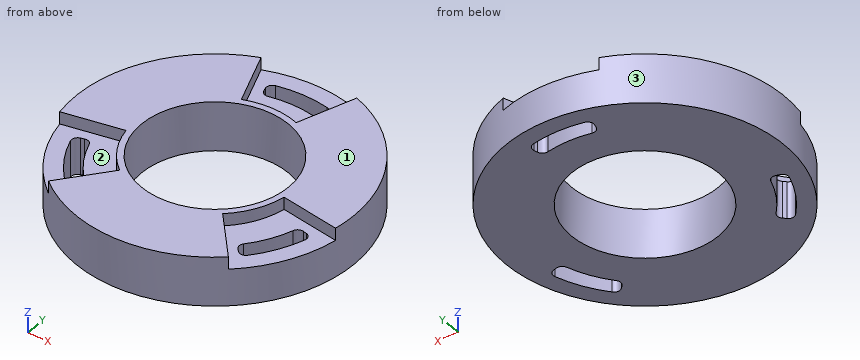
from build123d import *

# Parameters (mm, degrees)
CROQUIS1_R              = 11.35
CROQUIS1_R_2            = 6
SALIENTE_EXTRUIR1_DEPTH = 4
CORTAR_EXTRUIR1_START   = -1
CORTAR_EXTRUIR1_DEPTH   = 1


with BuildPart() as part:
    # Croquis1 → Saliente-Extruir1 (new body)
    with BuildSketch(Plane.XY):
        Circle(CROQUIS1_R)
        Circle(CROQUIS1_R_2, mode=Mode.SUBTRACT)
        with BuildLine():
            Line((2.377616051, 8.873383904), (2.455373053, 9.163576986))
            ThreePointArc((2.455373053, 9.163576986), (2.398691549, 9.55429889), (2.0762212, 9.782091061))
            ThreePointArc((2.0762212, 9.782091061), (0, 10), (-2.0762212, 9.782091061))
            ThreePointArc((-2.0762212, 9.782091061), (-2.398691549, 9.55429889), (-2.455373053, 9.163576986))
            Line((-2.455373053, 9.163576986), (-2.377616051, 8.873383904))
            ThreePointArc((-2.377616051, 8.873383904), (-2.15633175, 8.576736735), (-1.791682859, 8.513511175))
            ThreePointArc((-1.791682859, 8.513511175), (0, 8.7), (1.791682859, 8.513511175))
            ThreePointArc((1.791682859, 8.513511175), (2.15633175, 8.576736735), (2.377616051, 8.873383904))
        make_face(mode=Mode.SUBTRACT)
        with BuildLine():
            Line((8.873383904, -2.377616051), (9.163576986, -2.455373053))
            ThreePointArc((9.163576986, -2.455373053), (9.473611328, -2.699821628), (9.509649961, -3.092985228))
            ThreePointArc((9.509649961, -3.092985228), (8.660254038, -5), (7.433428761, -6.689105834))
            ThreePointArc((7.433428761, -6.689105834), (7.074919779, -6.854477262), (6.708203932, -6.708203932))
            Line((6.708203932, -6.708203932), (6.495767853, -6.495767853))
            ThreePointArc((6.495767853, -6.495767853), (6.34950602, -6.155806442), (6.477075524, -5.808398459))
            ThreePointArc((6.477075524, -5.808398459), (7.534421013, -4.35), (8.268758383, -2.705112716))
            ThreePointArc((8.268758383, -2.705112716), (8.505837769, -2.420930294), (8.873383904, -2.377616051))
        make_face(mode=Mode.SUBTRACT)
        with BuildLine():
            Line((-6.495767853, -6.495767853), (-6.708203932, -6.708203932))
            ThreePointArc((-6.708203932, -6.708203932), (-7.074919779, -6.854477262), (-7.433428761, -6.689105834))
            ThreePointArc((-7.433428761, -6.689105834), (-8.660254038, -5), (-9.509649961, -3.092985228))
            ThreePointArc((-9.509649961, -3.092985228), (-9.473611328, -2.699821628), (-9.163576986, -2.455373053))
            Line((-9.163576986, -2.455373053), (-8.873383904, -2.377616051))
            ThreePointArc((-8.873383904, -2.377616051), (-8.505837769, -2.420930294), (-8.268758383, -2.705112716))
            ThreePointArc((-8.268758383, -2.705112716), (-7.534421013, -4.35), (-6.477075524, -5.808398459))
            ThreePointArc((-6.477075524, -5.808398459), (-6.34950602, -6.155806442), (-6.495767853, -6.495767853))
        make_face(mode=Mode.SUBTRACT)
    extrude(amount=SALIENTE_EXTRUIR1_DEPTH)

    # Croquis2 → Cortar-Extruir1 (cut)
    with BuildSketch(Plane.XY.offset(4).offset(CORTAR_EXTRUIR1_START)):
        with BuildLine():
            Line((2.223130932, 6.108002035), (3.881928627, 10.665511246))
            ThreePointArc((3.881928627, 10.665511246), (0, 11.35), (-3.881928627, 10.665511246))
            Line((-3.881928627, 10.665511246), (-2.223130932, 6.108002035))
            ThreePointArc((-2.223130932, 6.108002035), (0, 6.5), (2.223130932, 6.108002035))
        make_face()
        with BuildLine():
            Line((6.401250395, -1.128713155), (11.177567997, -1.970906817))
            ThreePointArc((11.177567997, -1.970906817), (9.829388333, -5.675), (7.29563937, -8.694604429))
            Line((7.29563937, -8.694604429), (4.178119463, -4.97928888))
            ThreePointArc((4.178119463, -4.97928888), (5.629165125, -3.25), (6.401250395, -1.128713155))
        make_face()
        with BuildLine():
            Line((-4.178119463, -4.97928888), (-7.29563937, -8.694604429))
            ThreePointArc((-7.29563937, -8.694604429), (-9.829388333, -5.675), (-11.177567997, -1.970906817))
            Line((-11.177567997, -1.970906817), (-6.401250395, -1.128713155))
            ThreePointArc((-6.401250395, -1.128713155), (-5.629165125, -3.25), (-4.178119463, -4.97928888))
        make_face()
    extrude(amount=CORTAR_EXTRUIR1_DEPTH, mode=Mode.SUBTRACT)


solid = part.part
The listing builds one solid part. Answer for the finished solid, in the listing's coordinates (mm). Face numbers are marked on the shaded views. Coordinates: 2 decimals unless noted, no trailing zeros. Write each loop counter-clockwise with the first axis right and the second up, starting at its lowest first coordinate (ties: lowest second). Pieces come first, ordered by that corner, then holes. Notation, with made-up numbers: M 30,51 L 61,51 A31 cw 61,86 Z; hole C 85,-39 d10. An arc over 180 degrees is marked long. Put each result on its own line as item: value. Start each with the question number.
1. For a pull along Y with two mould halves and no side action, classify the marked faces 1, 2 and 3 as pulls with the +Y half, pulls with the -Y half, needs draft (parallel to the pull), parting line crosses it, or undercut.
2. A cutting plane is placed at C-C on y = 0. Write down the section's boundary in (x, z).
3. A cutting plane is placed at D-D on y = 5. Write down the section's boundary in (x, z).
4. Consider line 1 (Y direction, x = -2, z = 1.2); line 2 (Z direction, x = 2.25, y = 6.5); line 3 (Y direction, x = 9, z = 0.7). Determine where each line is inside the solid, lowest interval first. Write a range as from..to.
5. A cutting plane is placed at B-B on x = 0. Write down the section's boundary in (y, z).
6. Flat-ended cylindrical pins translate along their axes: P1, Ø1.5, axis at y = -3.5, z = 3, coming from the +X side; P2, Ø2, axis at y = 1.5, z = 1.5, coming from the +X side; P3, Ø1.6, axis at x = 1, y = 8, coming from the +Z side; P4, Ø7.5, axis at x = 8.5, y = -5, coming from the +Z side. Find the tip coordinate at first contact, or state that the pin passes through.
7. A cutting plane is placed at A-A on z = 3.5. Write down the section's boundary in (x, y).
Resolved:
1. face 1: needs draft
1. face 2: undercut
1. face 3: parting line crosses it
2. outline: M -11.35,0 L -6,0 L -6,4 L -11.35,4 Z; M 6,0 L 11.35,0 L 11.35,4 L 6,4 Z
3. outline: M -10.19,0 L -3.32,0 L -3.32,4 L -10.19,4 Z; M 3.32,0 L 10.19,0 L 10.19,4 L 3.32,4 Z
4. line 1: y = -11.17..-5.66, 5.66..8.51, 9.8..11.17
4. line 2: z = 0..3
4. line 3: y = -6.92..-4.36, -2.41..6.92
5. outline: M -11.35,0 L -6,0 L -6,4 L -11.35,4 Z; M 6,0 L 8.7,0 L 8.7,3 L 6.5,3 L 6.5,4 L 6,4 Z; M 10,0 L 11.35,0 L 11.35,3 L 10,3 Z
6. P1: stops at x = 11.01
6. P2: stops at x = 11.34
6. P3: stops at z = 3
6. P4: stops at z = 4
7. outline: M -11.18,-1.97 L -6.4,-1.13 A6.5 ccw -4.18,-4.98 L -7.3,-8.69 A11.35 ccw 7.3,-8.69 L 4.18,-4.98 A6.5 ccw 6.4,-1.13 L 11.18,-1.97 A11.35 ccw 3.88,10.67 L 2.22,6.11 A6.5 ccw -2.22,6.11 L -3.88,10.67 A11.35 ccw Z; hole C 0,0 d12
